Geometry check sheet. Reference: the model listing, model coordinates, mm. A direction names the side the tool comes from. Coordinates: 2 decimals unless noted, no trailing zeros. Loops run counter-clockwise (first coordinate to the right, second up) from the corner with the lowest first, then second, coordinate; pieces in that order, holes last.
from build123d import *

# Parameters (mm, degrees)
SKETCH1_W           = 254
SKETCH1_H           = 58.42
BOSS_EXTRUDE1_DEPTH = 19.05
CUT_EXTRUDE1_DEPTH  = 6.35
FILLET1_R           = 9.525
CUT_EXTRUDE2_START  = -127
SKETCH3_W           = 65.063506332
SKETCH3_H           = 25.722431086
CUT_EXTRUDE2_DEPTH  = 127
SKETCH4_R           = 2.54
BOSS_EXTRUDE2_DEPTH = 12.7
SKETCH5_W           = 12.7
SKETCH5_H           = 21.082
BOSS_EXTRUDE3_DEPTH = 6.35


with BuildPart() as part:
    # Sketch1 → Boss-Extrude1 (new body)
    with BuildSketch(Plane(origin=(0, 0, 0), x_dir=(1, 0, 0), z_dir=(0, 1, 0))):
        with Locations((127, 29.21)):
            Rectangle(SKETCH1_W, SKETCH1_H)
    extrude(amount=BOSS_EXTRUDE1_DEPTH)

    # Sketch2 → Cut-Extrude1 (cut)
    with BuildSketch(Plane(origin=(0, 19.05, 0), x_dir=(1, 0, 0), z_dir=(0, 1, 0))):
        Polygon((221.234, 52.07), (221.234, 18.288), (127, 18.288), (127, 0), (254, 0), (254, 58.42), (127, 58.42), (127, 52.07), align=None)
        Polygon((127, 0), (127, 18.288), (32.766, 18.288), (32.766, 52.07), (127, 52.07), (127, 58.42), (0, 58.42), (0, 0), align=None)
    extrude(amount=-CUT_EXTRUDE1_DEPTH, mode=Mode.SUBTRACT)

    # Fillet1
    fillet1_edges = [part.edges().sort_by_distance(p)[0] for p in [
        (254, 0, -29.21),
        (0, 0, -29.21),
    ]]
    fillet(fillet1_edges, radius=FILLET1_R)

    # Sketch3 → Cut-Extrude2 (cut)
    with BuildSketch(Plane.ZY.offset(CUT_EXTRUDE2_START)):
        with Locations((-32.531753166, 12.861215543)):
            Rectangle(SKETCH3_W, SKETCH3_H)
    extrude(amount=CUT_EXTRUDE2_DEPTH, mode=Mode.SUBTRACT)

    # Sketch4 → Boss-Extrude2 (add)
    with BuildSketch(Plane.ZY.offset(-127)):
        with Locations((-16.51, 6.35)):
            Circle(SKETCH4_R)
        with Locations((-29.21, 6.35)):
            Circle(SKETCH4_R)
        with Locations((-41.91, 6.35)):
            Circle(SKETCH4_R)
    extrude(amount=BOSS_EXTRUDE2_DEPTH)

    # Sketch5 → Boss-Extrude3 (add)
    with BuildSketch(Plane(origin=(0, 12.7, 0), x_dir=(1, 0, 0), z_dir=(0, 1, 0))):
        with Locations((227.584, 28.829)):
            Rectangle(SKETCH5_W, SKETCH5_H)
    extrude(amount=BOSS_EXTRUDE3_DEPTH)


solid = part.part
1) Section check C-C on y = 6.35. Record the cut outline in (x, z).
Data:
outline: (114.3, -44.45) - (127, -44.45) - (127, -58.42) - (253.46, -58.42) - (253.46, 0) - (127, 0) - (127, -13.97) - (114.3, -13.97) - (114.3, -19.05) - (127, -19.05) - (127, -26.67) - (114.3, -26.67) - (114.3, -31.75) - (127, -31.75) - (127, -39.37) - (114.3, -39.37) - close
2) Access from +Z, -Z, +X, -X, +Y, -Y to the whole of each face (thin tool, end or side, straight path). Record for faces 1 (the flat face through (173, 16, -52.07)), 2 (the flat face through (221.234, 16, -46)), 3 (the cylindrical face through (251.14, 2.72, -29.62)), 4 (the flat face through (233.934, 16, -29)), 5 (the cylindrical face through (120.739, 7.113, -39.487)).
Data:
face 1: -Z, +X, -X, +Y
face 2: -Z, +X, +Y
face 3: +Z, -Z, +X, -Y
face 4: +Z, -Z, +X, +Y
face 5: -X
3) Section check D-D on z = -46.5. Record the cut outline in (x, y) (3 decimals), and give its area (3 significant figures).
Data:
outline: (127, 0) - (244.475, 0) arc R9.525 ccw to (254, 9.525) - (254, 12.7) - (221.234, 12.7) - (221.234, 19.05) - (127, 19.05) - close
area: 2,190 mm2
4) Depth check by flat-ended pin: pin 1 (1.9 mm diameter, centred on x = 166, y = 15, fed in from -Z); pin 2 (2 mm diameter, centred on x = 173.5, y = 9, fed in from +Z); pin 3 (1 mm diameter, centred on y = 4.5, z = -43, fed in from +X); pin 4 (3 mm diameter, centred on x = 229, y = 17.5, fed in from -Z). Enter the tip coordinate at first touch or a pass-through.
Data:
pin 1: stops at z = -52.07
pin 2: stops at z = 0
pin 3: stops at x = 252.86
pin 4: stops at z = -39.37
5) Section check A-A on z = -20.5. Record the cut outline in (x, y) (3 decimals).
Data:
outline: (127, 0) - (244.475, 0) arc R9.525 ccw to (254, 9.525) - (254, 12.7) - (233.934, 12.7) - (233.934, 19.05) - (127, 19.05) - close
6) Section check B-B on x = 231. Record the cut outline in (y, z).
Data:
outline: (0, -58.42) - (12.7, -58.42) - (12.7, -39.37) - (19.05, -39.37) - (19.05, -18.29) - (12.7, -18.29) - (12.7, 0) - (0, 0) - close
7) Material ranges on probe 1 along Y at (x, z) = (239, -40); probe 2 along Z at (x, y) = (142, 12.75); probe 3 along X at (y, z) = (17, -20), recorded low to high.
Data:
probe 1: y = 0 to 12.7
probe 2: z = -52.07 to -18.29
probe 3: x = 127 to 233.93
8) Mould release check, pull along Z, two halves, no side actions. Record for faces 6 (the flat face through (180, 16, -18.288)), 7 (the flat face through (227, 16, -39.37)), 8 (the cylindrical face through (120.739, 7.113, -14.087)): +Z half, -Z half, draft (parallel to the pull), parting line (faces both ways), or undercut.
Data:
face 6: +Z half
face 7: -Z half
face 8: undercut
